from build123d import *

# Parameters (mm, degrees)
F0_R      = 12.5
F0_R_2    = 9.875
F1_DEPTH  = 4.95
F3_R      = 9.875
F3_R_2    = 9.625
F4_DEPTH  = 0.2
F6_R      = 9.875
F6_R_2    = 9.5
F7_DEPTH  = 0.4
F10_DEPTH = 0.4


with BuildPart() as f1:
    # F0 (on Top) → F1 (new body)
    with BuildSketch(Plane.XY):
        Circle(F0_R)
        Circle(F0_R_2, mode=Mode.SUBTRACT)
    extrude(amount=F1_DEPTH)

    # F3 (on offset) → F4 (join, symmetric)
    with BuildSketch(Plane.XY.offset(2.475)):
        Circle(F3_R)
        Circle(F3_R_2, mode=Mode.SUBTRACT)
    extrude(amount=F4_DEPTH, both=True)

    # F6 (on offset) → F7 (join)
    with BuildSketch(Plane(origin=(0, 0, 0), x_dir=(1, 0, 0), z_dir=(0, 0, -1))):
        Circle(F6_R)
        Circle(F6_R_2, mode=Mode.SUBTRACT)
    extrude(amount=-F7_DEPTH)

    # F9 (on offset) → F10 (join)
    with BuildSketch(Plane.XY.offset(4.95)):
        with BuildLine():
            ThreePointArc((0.125, -9.6241882775), (0, -9.625), (-0.125, -9.6241882775))
            Line((-0.125, -9.6241882775), (-0.125, -9.8742088291))
            ThreePointArc((-0.125, -9.8742088291), (0, -9.875), (0.125, -9.8742088291))
            Line((0.125, -9.8742088291), (0.125, -9.6241882775))
        make_face()
        with BuildLine():
            ThreePointArc((-0.125, -9.6241882775), (-6.7615641681, 6.8499543794), (9.625, 0))
            ThreePointArc((9.625, 0), (6.8499543794, -6.7615641681), (0.125, -9.6241882775))
            Line((0.125, -9.6241882775), (0.125, -9.8742088291))
            ThreePointArc((0.125, -9.8742088291), (7.0267346613, -6.9383445432), (9.875, 0))
            ThreePointArc((9.875, 0), (-6.9383445432, 7.0267346613), (-0.125, -9.8742088291))
            Line((-0.125, -9.8742088291), (-0.125, -9.6241882775))
        make_face()
    extrude(amount=-F10_DEPTH)


solid = f1.part
The listing builds one solid part. Answer for the finished solid, in the listing's coordinates (mm). A direction names the side the tool comes from. Coordinates: 2 decimals unless noted, no trailing zeros. Loops run counter-clockwise (first coordinate to the right, second up) from the corner with the lowest first, then second, coordinate; pieces in that order, holes last. Notation, with made-up numbers: (-27, -18.5) -> (11, -18.5) arc R20 cw to (11, 20.5) -> close; hole circle Ø8 at (-4.75, 78.25). An arc over 180 degrees is marked (long way). Answer in a Markdown table with one row per item. Add a question column.
1. The part is cut by section D-D, the plane y = 10.25. Write down the section's boundary in (x, z), then the cut area to 3 significant figures.
2. For faces 4 (the cylindrical face through (-7.28, 6.67, 1.32)), 5 (the cylindrical face through (-7.638, -5.857, 2.472)), 6 (the flat face through (2.7, -9.3, 0)), determine the directions among +Z, -Z, +X, -X, +Y, -Y from which every point of the face is accessible in a straight line to the end or side of a thin tool.
3. The part is cut by section A-A, the plane y = -2.5. Write down the section's boundary in (x, z) (3 decimals), then the cut area to 3 significant figures.
4. The part is cut by section B-B, the plane x = -6.75. Write down the section's boundary in (y, z) (3 decimals).
5. The part is cut by section C-C, the plane z = 4.2. Write down the section's boundary in (x, y) (3 decimals).
6. Determine the mould class of faces 1 (the cylindrical face through (9.419, 2.966, 3.599)), 2 (the flat face through (4, -9, 4.95)), 3 (the cylindrical face through (11.923, 3.755, 2.44)) for opening direction Z: +Z half, -Z half, draft (parallel to the pull), parting line (faces both ways), or undercut.
7. Consider line 1 (Y direction, x = 0, z = 4.7) (3 decimals); line 2 (Y direction, x = 0, z = 3.45) (3 decimals); line 3 (X direction, y = 5.25, z = 3.9). Determine where each line is inside the solid, lowest interval first. Write a range as [from, to].
8. Flat-ended cylindrical pins translate along their axes: P1, Ø1.5, axis at x = -6.5, z = 4, coming from the -Y side; P2, Ø1, axis at y = -9, z = 1, coming from the +X side. Find the tip coordinate at first contact, or state that the pin passes through.
Answer below:
| question | item | result |
|---|---|---|
| 1 | outline | (-7.15, 0) -> (7.15, 0) -> (7.15, 4.95) -> (-7.15, 4.95) -> close |
| 1 | area | 70.8 mm2 |
| 2 | face 4 | none |
| 2 | face 5 | +Z |
| 2 | face 6 | -Z, +X, -X, +Y, -Y |
| 3 | outline | (-12.247, 0) -> (-9.165, 0) -> (-9.165, 0.4) -> (-9.553, 0.4) -> (-9.553, 2.275) -> (-9.295, 2.275) -> (-9.295, 2.675) -> (-9.553, 2.675) -> (-9.553, 4.55) -> (-9.295, 4.55) -> (-9.295, 4.95) -> (-12.247, 4.95) -> close; (9.165, 0) -> (12.247, 0) -> (12.247, 4.95) -> (9.295, 4.95) -> (9.295, 4.55) -> (9.553, 4.55) -> (9.553, 2.675) -> (9.295, 2.675) -> (9.295, 2.275) -> (9.553, 2.275) -> (9.553, 0.4) -> (9.165, 0.4) -> close |
| 3 | area | 27.4 mm2 |
| 4 | outline | (-10.521, 0) -> (-6.685, 0) -> (-6.685, 0.4) -> (-7.208, 0.4) -> (-7.208, 2.275) -> (-6.861, 2.275) -> (-6.861, 2.675) -> (-7.208, 2.675) -> (-7.208, 4.55) -> (-6.861, 4.55) -> (-6.861, 4.95) -> (-10.521, 4.95) -> close; (6.685, 0) -> (10.521, 0) -> (10.521, 4.95) -> (6.861, 4.95) -> (6.861, 4.55) -> (7.208, 4.55) -> (7.208, 2.675) -> (6.861, 2.675) -> (6.861, 2.275) -> (7.208, 2.275) -> (7.208, 0.4) -> (6.685, 0.4) -> close |
| 5 | outline | circle Ø25 at (0, 0); hole circle Ø19.75 at (0, 0) |
| 6 | face 1 | undercut |
| 6 | face 2 | +Z half |
| 6 | face 3 | draft |
| 7 | line 1 | [-12.5, -9.625], [9.625, 12.5] |
| 7 | line 2 | [-12.5, -9.875], [9.875, 12.5] |
| 7 | line 3 | [-11.34, -8.36], [8.36, 11.34] |
| 8 | P1 | y = -11.1 |
| 8 | P2 | x = 9.17 |
